The model under review builds one solid part; all positions refer to its coordinate system, in mm. Face numbers are marked on the shaded views. Coordinates: 2 decimals unless noted, no trailing zeros. Order: outer loops, then holes, each group sorted by start corner. A loop starts at its lowest first (then second) coordinate and runs counter-clockwise, first axis right, second up. Notation, with made-up numbers: M 64,33 L 86,33 A19 cw 86,41 Z; hole C 25.25,68 d7. An arc over 180 degrees is marked long. Answer as CSV lines item,"result". Start each with the question number.
Q1. Consider section A-A on y = 30. Write out the cut boundary in (x, z).
Q2. Consider section D-D on x = -4. Write out the cut boundary in (y, z).
Q3. For P1, Ø8, axis at x = -16, y = 50, coming from the +Z side, flat-tipped, find the tip position at first contact; note if it passes through.
Q4. Wall thickness on L1, parallel to Y at x = -55, z = 14.5; L2, parallel to Y at x = -30, z = 8; L3, parallel to X at y = 47, z = 13.75: over which ranges is each line inside the solid? List them lowest first. Write a range as [from, to].
Q5. Consider section C-C on z = 21. Write out the cut boundary in (x, y), and give its area (3 significant figures).
Q6. The part is to be moulded in two halves that separate along X. For the marked faces 1, 2 and 3, say which applies: +X half, -X half, draft (parallel to the pull), parting line (faces both ways), or undercut.
Q7. Consider section B-B on x = -30. Write out the cut boundary in (y, z), and give its area (3 significant figures).
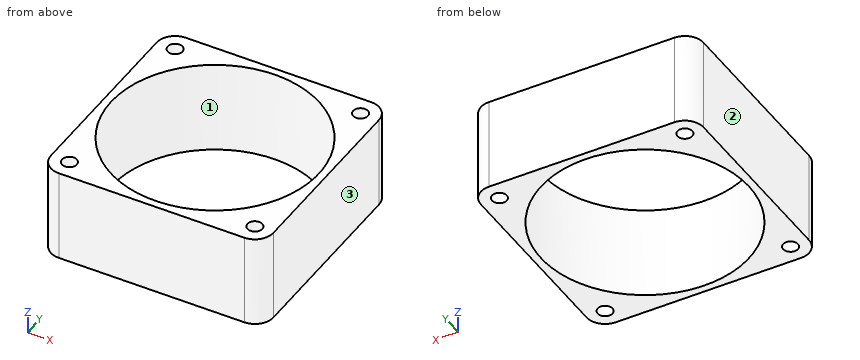
from build123d import *

# Parameters (mm, degrees)
ESQUISSE1_W             = 60
ESQUISSE1_H             = 60
BOSS_EXTRU_1_DEPTH      = 25
ENL_V_MAT_EXTRU_1_REACH = 27
ESQUISSE2_R             = 28
ESQUISSE3_R             = 2
ENL_V_MAT_EXTRU_2_DEPTH = 25
CONG_1_R                = 5


with BuildPart() as part:
    # Esquisse1 → Boss.-Extru.1 (new body)
    with BuildSketch(Plane.XY):
        with Locations((-30, 30)):
            Rectangle(ESQUISSE1_W, ESQUISSE1_H)
    extrude(amount=BOSS_EXTRU_1_DEPTH)

    # Esquisse2 → Enl_v. mat.-Extru.1 (cut, up to next)
    with BuildSketch(Plane(origin=(0, 0, 0), x_dir=(-1, 0, 0), z_dir=(0, 0, -1)), mode=Mode.PRIVATE) as enl_v_mat_extru_1_sk1:
        with Locations((30, 30)):
            Circle(ESQUISSE2_R)
    enl_v_mat_extru_1_tool1 = extrude(enl_v_mat_extru_1_sk1.sketch, amount=-ENL_V_MAT_EXTRU_1_REACH, mode=Mode.PRIVATE) & part.part
    add(enl_v_mat_extru_1_tool1.solids().sort_by_distance((-30, 30, 0))[0], mode=Mode.SUBTRACT)

    # Esquisse3 → Enl_v. mat.-Extru.2 (cut)
    with BuildSketch(Plane(origin=(0, 0, 0), x_dir=(-1, 0, 0), z_dir=(0, 0, -1))):
        with Locations((5, 55)):
            Circle(ESQUISSE3_R)
        with Locations((55, 55)):
            Circle(ESQUISSE3_R)
        with Locations((55, 5)):
            Circle(ESQUISSE3_R)
        with Locations((5, 5)):
            Circle(ESQUISSE3_R)
    extrude(amount=-ENL_V_MAT_EXTRU_2_DEPTH, mode=Mode.SUBTRACT)

    # Cong_1
    cong_1_edges = [part.edges().sort_by_distance(p)[0] for p in [
        (-60, 60, 12.5),
        (0, 60, 12.5),
        (0, 0, 12.5),
        (-60, 0, 12.5),
    ]]
    fillet(cong_1_edges, radius=CONG_1_R)


solid = part.part
Evaluation:
1,outline,"M -60,0 L -58,0 L -58,25 L -60,25 Z; M -2,0 L 0,0 L 0,25 L -2,25 Z"
2,outline,"M 0.1,0 L 3.27,0 L 3.27,25 L 0.1,25 Z; M 6.73,0 L 19.61,0 L 19.61,25 L 6.73,25 Z; M 40.39,0 L 53.27,0 L 53.27,25 L 40.39,25 Z; M 56.73,0 L 59.9,0 L 59.9,25 L 56.73,25 Z"
3,P1,"stops at z = 25"
4,L1,"y = [0, 3], [7, 17.39], [42.61, 53], [57, 60]"
4,L2,"y = [0, 2], [58, 60]"
4,L3,"x = [-60, -52.25], [-7.75, 0]"
5,outline,"M -60,5 A5 ccw -55,0 L -5,0 A5 ccw 0,5 L 0,55 A5 ccw -5,60 L -55,60 A5 ccw -60,55 Z; hole C -30,30 d56; hole C -55,5 d4; hole C -55,55 d4; hole C -5,5 d4; hole C -5,55 d4"
5,area,"1,070 mm²"
6,face 1,"undercut"
6,face 2,"-X half"
6,face 3,"+X half"
7,outline,"M 0,0 L 2,0 L 2,25 L 0,25 Z; M 58,0 L 60,0 L 60,25 L 58,25 Z"
7,area,"100 mm²"
